from build123d import *

# Parameters (mm, degrees)
F1_DEPTH  = 30
F2_R      = 3.75
F3_DEPTH  = 30
F4_W      = 30.0004304858
F4_H      = 9
F5_DEPTH  = 42
F6_SIZE   = 5
F7_W      = 0.0346347876
F7_H      = 6.4651286568
F8_DEPTH  = 21
F10_DEPTH = 25


with BuildPart() as f1:
    # F0 (on Top) → F1 (new body)
    with BuildSketch(Plane.XY):
        with BuildLine():
            Line((8.7358052025, -10.7137067538), (8.5750901289, 19.2862932462))
            Line((8.5750901289, 19.2862932462), (-9.4249098711, 19.2862932462))
            ThreePointArc((-9.4249098711, 19.2862932462), (-24.3445523343, 4.2059357094), (-9.2641947975, -10.7137067538))
            Line((-9.2641947975, -10.7137067538), (8.7358052025, -10.7137067538))
        make_face()
    extrude(amount=F1_DEPTH)

    # F2 (on face) → F3 (cut)
    with BuildSketch(Plane.XY.offset(30)):
        with Locations((-4.9572857097, 4.1074641049)):
            Circle(F2_R)
    extrude(amount=-F3_DEPTH, mode=Mode.SUBTRACT)

    # F4 (on face) → F5 (join)
    with BuildSketch(Plane(origin=(8.6781610067, 0.0464903762, 0), x_dir=(-0.0053570922, 0.9999856507, 0), z_dir=(0.9999856507, 0.0053570922, 0))):
        with Locations((4.2398637092, 4.5)):
            Rectangle(F4_W, F4_H)
    extrude(amount=F5_DEPTH)

    # F6
    f6_edges = [f1.edges().sort_by_distance(p)[0] for p in [
        (50.735203, -10.488709, 4.5),
        (50.574487, 19.511291, 4.5),
    ]]
    chamfer(f6_edges, length=F6_SIZE)

    # F7 (on face) → F8 (join)
    with BuildSketch(Plane.XY.offset(9)):
        with Locations((50.6616953499, 3.2325643284)):
            Rectangle(F7_W, F7_H)
        Polygon((8.6409098797, 0), (50.6443779561, 0), (50.6443779561, 6.4651286568), (50.6790127437, 6.4651286568), (50.6790127437, 7), (8.6409098797, 7), align=None)
    extrude(amount=F8_DEPTH)

    # F9 (on face) → F10 (cut)
    with BuildSketch(Plane.XZ):
        Polygon((50.6790127437, 30), (8.6784100635, 30), (50.6790127437, 9), align=None)
    extrude(amount=-F10_DEPTH, mode=Mode.SUBTRACT)


solid = f1.part
Build history of the part. All positions in model axes, mm. A direction names the side the tool comes from. Coordinates: 2 decimals unless noted, no trailing zeros. Order: outer loops, then holes, each group sorted by start corner. A loop starts at its lowest first (then second) coordinate and runs counter-clockwise, first axis right, second up. Notation, with made-up numbers: (59, 79) -> (110, 79) arc R15 cw to (110, 99) -> close; hole circle Ø8 at (6, 5.25). An arc over 180 degrees is marked (long way). One line per item, written item: value.
(1) Mould opens along X. For faces 1 (the flat face through (0, 19.286, 15)), 2 (the cylindrical face through (-5.77, 0.447, 15.21)), 3 (the flat face through (29.38, 3.45, 19.65)) say: pulls with the +X half, pulls with the -X half, needs draft (parallel to the pull), parting line crosses it, or undercut.
Checked values:
face 1: needs draft
face 2: undercut
face 3: pulls with the +X half
(2) Tool access for faces 4 (the flat face through (25, 7, 17)), 5 (the flat face through (29, -5, 9)), 6 (the flat face through (48.053, 17.033, 4.437)): list every direction of +Z, -Z, +X, -X, +Y, -Y with a clear straight run to the whole face (end or side of a thin tool).
Checked values:
face 4: +Z, +X, +Y
face 5: +Z, +X, -Y
face 6: +Z, -Z, +X, +Y
(3) Slice it at C-C, the plane x = 34.5. List the corners of the cut face in (y, z).
Checked values:
outline: (-10.58, 0) -> (19.43, 0) -> (19.43, 9) -> (7, 9) -> (7, 17.09) -> (0, 17.09) -> (0, 9) -> (-10.58, 9) -> close
(4) Drop flat-ended pins along their axis: pin 1 Ø1.5 at (y, z) = (15.5, 5.5) entering from -X; pin 2 Ø8 at (y, z) = (-3.5, 13) entering from -X; pin 3 Ø14.5 at (x, z) = (-2.5, 21.5) entering from +Y. Give the stop position or say it passes through.
Checked values:
pin 1: x = -20.09
pin 2: x = -23.86
pin 3: y = 19.29
(5) Slice it at D-D, the plane z = 20.25. List the corners of the cut face in (x, y).
Checked values:
outline: (-9.42, 19.29) arc R15 ccw to (-9.26, -10.71) -> (8.74, -10.71) -> (8.68, 0) -> (28.18, 0) -> (28.18, 7) -> (8.64, 7) -> (8.58, 19.29) -> close; hole circle Ø7.5 at (-4.96, 4.11)
(6) Slice it at A-A, the plane z = 11.75. List the corners of the cut face in (x, y).
Checked values:
outline: (-9.42, 19.29) arc R15 ccw to (-9.26, -10.71) -> (8.74, -10.71) -> (8.68, 0) -> (45.18, 0) -> (45.18, 7) -> (8.64, 7) -> (8.58, 19.29) -> close; hole circle Ø7.5 at (-4.96, 4.11)
(7) Probe line 1 (Y direction, x = 35, z = 13.75); line 2 (Y direction, x = 0, z = 17.5); line 3 (Z direction, x = 18.5, y = -3). List the from-to ranges inside material, lowest first. Write a range as [from, to].
Checked values:
line 1: [0, 7]
line 2: [-10.71, 19.29]
line 3: [0, 9]
